```python
from build123d import *

# Parameters (mm, degrees)
RESSALTO_EXTRUS_O1_DEPTH = 8.6
ESBO_O2_R                = 0.9
CORTE_EXTRUS_O1_DEPTH    = 15
ESBO_O3_R                = 4.3
ESBO_O3_R_2              = 2.4
RESSALTO_EXTRUS_O3_DEPTH = 4.6
ESBO_O4_R                = 1.9
ESBO_O4_R_2              = 0.75
RESSALTO_EXTRUS_O4_DEPTH = 3
RESSALTO_EXTRUS_O5_DEPTH = 3
PADR_OCIRCULAR1_COUNT    = 24


with BuildPart() as part:
    # Esboço1 → Ressalto-extrusão1 (new body)
    with BuildSketch(Plane.XY):
        Polygon((0, 0), (0, 13), (-5.5, 13), (-5.5, 14), (0, 14), (0, 17.4), (19.65, 17.4), (19.65, 14), (25.15, 14), (25.15, 13), (19.65, 13), (19.65, 0), align=None)
    extrude(amount=RESSALTO_EXTRUS_O1_DEPTH)

    # Esboço2 → Corte-extrusão1 (cut, through all)
    with BuildSketch(Plane(origin=(0, 14, 0), x_dir=(1, 0, 0), z_dir=(0, 1, 0))):
        with Locations((-3, -4.3)):
            Circle(ESBO_O2_R)
        with Locations((22.65, -4.3)):
            Circle(ESBO_O2_R)
    extrude(amount=-CORTE_EXTRUS_O1_DEPTH, mode=Mode.SUBTRACT)

    # Esboço3 → Ressalto-extrusão3 (add)
    with BuildSketch(Plane(origin=(0, 17.4, 0), x_dir=(1, 0, 0), z_dir=(0, 1, 0))):
        with Locations((4.3, -4.3)):
            Circle(ESBO_O3_R)
        with Locations((8.5, -4.3)):
            Circle(ESBO_O3_R_2)
    extrude(amount=RESSALTO_EXTRUS_O3_DEPTH)

    # Esboço4 → Ressalto-extrusão4 (add)
    with BuildSketch(Plane(origin=(0, 22, 0), x_dir=(1, 0, 0), z_dir=(0, 1, 0))):
        with Locations((4.3, -4.3)):
            Circle(ESBO_O4_R)
        with Locations((4.3, -4.3)):
            Circle(ESBO_O4_R_2, mode=Mode.SUBTRACT)
    extrude(amount=RESSALTO_EXTRUS_O4_DEPTH)

    # Esboço5 → Ressalto-extrusão5 (add)
    with BuildSketch(Plane(origin=(0, 25, 0), x_dir=(1, 0, 0), z_dir=(0, 1, 0))):
        with BuildLine():
            Line((3.996143779, -2.424454374), (4.147072388, -2.164733177))
            ThreePointArc((4.147072388, -2.164733177), (4.320558883, -2.065222191), (4.493481171, -2.16571041))
            Line((4.493481171, -2.16571041), (4.646102398, -2.431788789))
            Line((4.646102398, -2.431788789), (3.996143779, -2.424454374))
        make_face()
    ressalto_extrus_o5 = extrude(amount=-RESSALTO_EXTRUS_O5_DEPTH)

    # PadrãoCircular1: Ressalto-extrusão5 ×24 about axis
    padr_ocircular1_axis = Axis((4.3, 0, 4.3), (0, 1, 0))
    for i in range(1, PADR_OCIRCULAR1_COUNT):
        add(ressalto_extrus_o5.rotate(padr_ocircular1_axis, i * 360 / PADR_OCIRCULAR1_COUNT))


solid = part.part
```
Geometry: final body of the model. Coordinates: model frame, mm. A direction names the side the tool comes from. Coordinates: 2 decimals unless noted, no trailing zeros. Order: outer loops, then holes, each group sorted by start corner. A loop starts at its lowest first (then second) coordinate and runs counter-clockwise, first axis right, second up.
Item 1: Section query C-C (z = 1). Output: boundary loops of the cut face in (x, y).
Answer:
outline: (-5.5, 13) - (0, 13) - (0, 0) - (19.65, 0) - (19.65, 13) - (25.15, 13) - (25.15, 14) - (19.65, 14) - (19.65, 17.4) - (7.06, 17.4) - (7.06, 22) - (1.54, 22) - (1.54, 17.4) - (0, 17.4) - (0, 14) - (-5.5, 14) - close
Item 2: Section query A-A (x = -3). Output: boundary loops of the cut face in (y, z), then the cut area to 3 significant figures.
Answer:
outline: (13, 0) - (14, 0) - (14, 3.4) - (13, 3.4) - close; (13, 5.2) - (14, 5.2) - (14, 8.6) - (13, 8.6) - close
area: 6.80 mm2
Item 3: Draft query along X for faces 1 (the face through (4, 22, 4)), 2 (the face through (1, 17.4, 8)), 3 (the face through (19.65, 7, 4)). Return one class per face: released by +X, released by -X, zero draft, split by the parting line, or undercut.
Answer:
face 1: undercut
face 2: zero draft
face 3: released by +X
Item 4: Access query for faces 4 (the face through (7, 22, 4)), 5 (the face through (1, 17.4, 1)), 6 (the face through (0, 16, 4)), 7 (the face through (22, 13, 3)). Directions: +Z, -Z, +X, -X, +Y, -Y. A direction counts if a zero-diameter tool reaches every point of the face in a straight line with its end or side. Return the directions, or none.
Answer:
face 4: +Y
face 5: -Z, -X, +Y
face 6: +Z, -Z, -X, +Y
face 7: +Z, -Z, +X, -Y
Item 5: Section query D-D (y = 5). Output: boundary loops of the cut face in (x, z), then the cut area to 3 significant figures.
Answer:
outline: (0, 0) - (19.65, 0) - (19.65, 8.6) - (0, 8.6) - close
area: 169 mm2
Item 6: Contact query for flat-ended pins moving along their axis: P1, Ø3, axis at x = -3, z = 4.3, coming from the +Y side; P2, Ø1, axis at y = 15.5, z = 6, coming from the +X side; P3, Ø4.5, axis at x = 10.5, z = 5, coming from the +Y side. Output: stop coordinate, or through.
Answer:
P1: stops at y = 14
P2: stops at x = 19.65
P3: stops at y = 22
Item 7: Section query B-B (x = 8.5). Output: boundary loops of the cut face in (y, z), then the cut area to 3 significant figures.
Answer:
outline: (0, 0) - (17.4, 0) - (17.4, 1.9) - (22, 1.9) - (22, 6.7) - (17.4, 6.7) - (17.4, 8.6) - (0, 8.6) - close
area: 172 mm2
Item 8: Material intervals for line 1 along X through (y, z) = (13.65, 4.3); line 2 along Z through (x, y) = (4.3, 23.85); line 3 along Z through (x, y) = (-3, 13.75), sorted ascending.
Answer:
line 1: x = -5.5 to -3.9, -2.1 to 21.75, 23.55 to 25.15
line 2: z = 2.07 to 3.55, 5.05 to 6.53
line 3: z = 0 to 3.4, 5.2 to 8.6
